```python
from build123d import *

# Parameters (mm, degrees)
SKETCH1_R           = 50
BOSS_EXTRUDE1_DEPTH = 120
SHELL1_T            = -3
SKETCH2_R           = 4
BOSS_EXTRUDE2_DEPTH = 5


with BuildPart() as part:
    # Sketch1 → Boss-Extrude1 (new body)
    with BuildSketch(Plane(origin=(0, 0, 0), x_dir=(1, 0, 0), z_dir=(0, 1, 0))):
        with Locations(Location((0, 0, 0), (0, 0, 270))):
            Circle(SKETCH1_R)
    extrude(amount=BOSS_EXTRUDE1_DEPTH)

    # Shell1
    shell1_openings = [part.faces().sort_by_distance(p)[0] for p in [
        (0, 120, 0),
    ]]
    offset(amount=SHELL1_T, openings=shell1_openings, kind=Kind.INTERSECTION)

    # Sketch2 → Boss-Extrude2 (add)
    with BuildSketch(Plane.XZ):
        with BuildLine():
            Line((49.434299833, 7.5), (65, 7.5))
            Line((65, 7.5), (65, -7.5))
            Line((65, -7.5), (49.434299833, -7.5))
            ThreePointArc((49.434299833, -7.5), (50, 0), (49.434299833, 7.5))
        make_face()
        with Locations(Location((57, 0, 0), (0, 0, 270))):
            Circle(SKETCH2_R, mode=Mode.SUBTRACT)
        with BuildLine():
            Line((-18.221959388, -46.561359474), (-26.004809472, -60.041651246))
            Line((-26.004809472, -60.041651246), (-38.995190528, -52.541651246))
            Line((-38.995190528, -52.541651246), (-31.212340445, -39.061359474))
            ThreePointArc((-31.212340445, -39.061359474), (-25, -43.301270189), (-18.221959388, -46.561359474))
        make_face()
        with Locations(Location((-28.5, -49.363448016, 0), (0, 0, 270))):
            Circle(SKETCH2_R, mode=Mode.SUBTRACT)
        with BuildLine():
            Line((-31.212340445, 39.061359474), (-38.995190528, 52.541651246))
            Line((-38.995190528, 52.541651246), (-26.004809472, 60.041651246))
            Line((-26.004809472, 60.041651246), (-18.221959388, 46.561359474))
            ThreePointArc((-18.221959388, 46.561359474), (-25, 43.301270189), (-31.212340445, 39.061359474))
        make_face()
        with Locations(Location((-28.5, 49.363448016, 0), (0, 0, 270))):
            Circle(SKETCH2_R, mode=Mode.SUBTRACT)
    extrude(amount=-BOSS_EXTRUDE2_DEPTH)


solid = part.part
```
Could you check a few things on this model? Use its own coordinates, in mm. A direction names the side the tool comes from. Coordinates: 2 decimals unless noted, no trailing zeros. Write each loop counter-clockwise with the first axis right and the second up, starting at its lowest first coordinate (ties: lowest second). Pieces come first, ordered by that corner, then holes. Notation, with made-up numbers: (13.25, -10) - (25.25, -10) arc R22 cw to (25.25, 8) - close; hole circle Ø10 at (-37, 1.5). An arc over 180 degrees is marked (long way). Use a Markdown table: item, result.
Q1. Which directions (+Z, -Z, +X, -X, +Y, -Y) give clear straight access to the entire face, cutting with the end or side of a thin tool? Please do faces 5 (the flat face through (-33, 5, -49)), 6 (the flat face through (-33, 5, 50)), 7 (the flat face through (57, 2, 7.5)), 8 (the cylindrical face through (15.02, 59.16, 47.69)).
Geometry check:
| item | result |
|---|---|
| face 5 | -Z, -X, +Y |
| face 6 | +Z, -X, +Y |
| face 7 | +Z, +X, +Y, -Y |
| face 8 | +Y |
Q2. Thinking about a two-plate mould opening in X: for faces 1 (the flat face through (-22.06, 2.46, -53.21)), 2 (the flat face through (61, 5, 2)), 3 (the cylindrical face through (-28.324, 2.465, -45.367)), 4 (the flat face through (-35.05, 2.46, 45.71)), which applies, +X half, -X half, draft (parallel to the pull), parting line (faces both ways), or undercut?
Geometry check:
| item | result |
|---|---|
| face 1 | undercut |
| face 2 | draft |
| face 3 | undercut |
| face 4 | -X half |
Q3. I'm going to push flat-ended pins straight in: pin 1 Ø8 at (x, z) = (7, 27.5) entering from -Y; pin 2 Ø5 at (y, z) = (105.5, 1.5) entering from -X; pin 3 Ø6.5 at (x, z) = (-28.5, 49.36) entering from -Y; pin 4 Ø2.5 at (x, y) = (56.5, 3) entering from -Z. Where does each tip first touch, or does it pass through?
Geometry check:
| item | result |
|---|---|
| pin 1 | stops at y = 0 |
| pin 2 | stops at x = -50 |
| pin 3 | passes through |
| pin 4 | stops at z = -7.5 |
Q4. Please list where these lines run through material, in increasing order: L1, parallel to X at y = 3.6, z = 0; L2, parallel to Z at x = 0, y = 34.
Geometry check:
| item | result |
|---|---|
| L1 | x = -50 to -47, 47 to 53, 61 to 65 |
| L2 | z = -50 to -47, 47 to 50 |
Q5. Imagine slicing it at C-C (x = -35.5). List the corners of the cut face in (y, z) for me.
Geometry check:
| item | result |
|---|---|
| outline | (0, -54.56) - (5, -54.56) - (5, -46.49) - (0, -46.49) - close; (0, -35.21) - (120, -35.21) - (120, -30.8) - (3, -30.8) - (3, 30.8) - (120, 30.8) - (120, 35.21) - (0, 35.21) - close; (0, 46.49) - (5, 46.49) - (5, 54.56) - (0, 54.56) - close |
Q6. Imagine slicing it at D-D (y = 55). List the corners of the cut face in (x, z) for me, and give its area (3 significant figures).
Geometry check:
| item | result |
|---|---|
| outline | circle Ø100 at (0, 0); hole circle Ø94 at (0, 0) |
| area | 914 mm2 |
Q7. Imagine slicing it at A-A (x = 57). List the corners of the cut face in (y, z) for me.
Geometry check:
| item | result |
|---|---|
| outline | (0, -7.5) - (5, -7.5) - (5, -4) - (0, -4) - close; (0, 4) - (5, 4) - (5, 7.5) - (0, 7.5) - close |
Q8. Imagine slicing it at B-B (z = 0). List the corners of the cut face in (x, y) for me, and give its area (3 significant figures).
Geometry check:
| item | result |
|---|---|
| outline | (-50, 0) - (53, 0) - (53, 5) - (50, 5) - (50, 120) - (47, 120) - (47, 3) - (-47, 3) - (-47, 120) - (-50, 120) - close; (61, 0) - (65, 0) - (65, 5) - (61, 5) - close |
| area | 1,040 mm2 |
